Verification items for the finished model (mm, model axes). Round coordinates to 2 decimals unless told otherwise and drop trailing zeros. Order: outer loops, then holes, each group sorted by start corner. A loop starts at its lowest first (then second) coordinate and runs counter-clockwise, first axis right, second up. Notation, with made-up numbers: (47.25, -16) -> (60.25, -16) arc R6 cw to (60.25, -8) -> close; hole circle Ø2 at (37.5, 70). An arc over 180 degrees is marked (long way). Put each result on its own line as item: value.
from build123d import *

# Parameters (mm, degrees)
SKETCH1_W            = 50.8
SKETCH1_H            = 4.7752
BOSS_EXTRUDE1_DEPTH  = 38.1
CUT_EXTRUDE2_DEPTH   = 7.62
SKETCH9_R            = 3.151882158
CUT_EXTRUDE3_DEPTH   = 47.038815526
LPATTERN1_COUNT      = 3
LPATTERN1_PITCH      = 25.4
LPATTERN1_COUNT_DIR2 = 2
LPATTERN1_PITCH_DIR2 = 25.4


with BuildPart() as part:
    # Sketch1 → Boss-Extrude1 (new, symmetric)
    with BuildSketch(Plane.XY):
        Rectangle(SKETCH1_W, SKETCH1_H)
    extrude(amount=BOSS_EXTRUDE1_DEPTH, both=True)

    # Sketch8 → Cut-Extrude2 (cut)
    with BuildSketch(Plane(origin=(0, 2.3876, 0), x_dir=(-1, 0, 0), z_dir=(0, 1, 0))):
        Polygon((0, -38.1), (-25.4, 12.7), (-25.4, -38.1), align=None)
    extrude(amount=-CUT_EXTRUDE2_DEPTH, mode=Mode.SUBTRACT)

    # Sketch9 → Cut-Extrude3 (cut, through all)
    with BuildSketch(Plane(origin=(0, 2.3876, 0), x_dir=(1, 0, 0), z_dir=(0, 1, 0))):
        with Locations(Location((-12.7, 25.4, 0), (0, 0, 270))):
            Circle(SKETCH9_R)
    cut_extrude3 = extrude(amount=-CUT_EXTRUDE3_DEPTH, mode=Mode.SUBTRACT)

    # LPattern1: Cut-Extrude3 3 × 2, 2 skipped
    with Locations(*[(j * LPATTERN1_PITCH_DIR2, 0, i * LPATTERN1_PITCH) for i in range(LPATTERN1_COUNT) for j in range(LPATTERN1_COUNT_DIR2) if (i, j) not in ((0, 0), (0, 1), (1, 1))]):
        add(cut_extrude3, mode=Mode.SUBTRACT)


solid = part.part
Item 1: Material ranges on L1, parallel to X at y = -0.6, z = 25.4; L2, parallel to Z at x = -15, y = 0.95; L3, parallel to Z at x = -10, y = 2.2, recorded low to high. Write a range as [from, to].
Check sheet entries:
L1: x = [-25.4, -15.85], [-9.55, 9.55], [15.85, 25.4]
L2: z = [-38.1, -27.56], [-23.24, -2.16], [2.16, 23.24], [27.56, 38.1]
L3: z = [-38.1, -27.03], [-23.77, -1.63], [1.63, 23.77], [27.03, 38.1]
Item 2: Section check B-B on z = 0. Record the boundary of the cut face in (x, y).
Check sheet entries:
outline: (-25.4, -2.39) -> (-15.85, -2.39) -> (-15.85, 2.39) -> (-25.4, 2.39) -> close; (-9.55, -2.39) -> (19.05, -2.39) -> (19.05, 2.39) -> (-9.55, 2.39) -> close
Item 3: Gauge pin test, flat end, axial feed: pin 1 Ø5.5 at (x, z) = (-12.7, 0) entering from -Y. Record the tip position at first contact, or that the pin passes through.
Check sheet entries:
pin 1: passes through
Item 4: Release check for a two-part mould opening along X. For faces 1 (the flat face through (-25.4, 0, 1)), 2 (the flat face through (25.4, 0, 26)), 3 (the flat face through (-6, 2.388, 1)), 4 (the cylindrical face through (-15.777, 0.033, -0.683)) record: +X half, -X half, draft (parallel to the pull), parting line (faces both ways), or undercut.
Check sheet entries:
face 1: -X half
face 2: +X half
face 3: draft
face 4: undercut
Item 5: Section check A-A on x = 12.7. Record the boundary of the cut face in (y, z), then the cut area to 3 significant figures.
Check sheet entries:
outline: (-2.39, -12.7) -> (2.39, -12.7) -> (2.39, 22.25) -> (-2.39, 22.25) -> close; (-2.39, 28.55) -> (2.39, 28.55) -> (2.39, 38.1) -> (-2.39, 38.1) -> close
area: 212 mm^2
Item 6: Section check C-C on y = -1. Record the boundary of the cut face in (x, z).
Check sheet entries:
outline: (-25.4, -38.1) -> (0, -38.1) -> (25.4, 12.7) -> (25.4, 38.1) -> (-25.4, 38.1) -> close; hole circle Ø6.3 at (-12.7, -25.4); hole circle Ø6.3 at (-12.7, 0); hole circle Ø6.3 at (-12.7, 25.4); hole circle Ø6.3 at (12.7, 25.4)
Item 7: Section check D-D on z = 25.4. Record the boundary of the cut face in (x, y).
Check sheet entries:
outline: (-25.4, -2.39) -> (-15.85, -2.39) -> (-15.85, 2.39) -> (-25.4, 2.39) -> close; (-9.55, -2.39) -> (9.55, -2.39) -> (9.55, 2.39) -> (-9.55, 2.39) -> close; (15.85, -2.39) -> (25.4, -2.39) -> (25.4, 2.39) -> (15.85, 2.39) -> close
